Verification items for the finished model (mm, model axes). A direction names the side the tool comes from. Round coordinates to 2 decimals unless told otherwise and drop trailing zeros. Order: outer loops, then holes, each group sorted by start corner. A loop starts at its lowest first (then second) coordinate and runs counter-clockwise, first axis right, second up. Notation, with made-up numbers: (89.25, -11) -> (140.25, -11) arc R30 cw to (140.25, 14) -> close; hole circle Ø9 at (81.5, -12.5). An arc over 180 degrees is marked (long way). Answer in a Markdown table with one row per item. Add a question column.
```python
from build123d import *

# Parameters (mm, degrees)
F0_R     = 1.1684
F1_DEPTH = 4.5085
F3_DEPTH = 4.953
F5_DEPTH = 4.4069
F6_R     = 0.254
F7_DEPTH = 3.81


with BuildPart() as f1:
    # F0 (on Top) → F1 (new body, symmetric)
    with BuildSketch(Plane.XY):
        with BuildLine():
            Line((8.3947, 3.937), (-8.3947, 3.937))
            ThreePointArc((-8.3947, 3.937), (-9.508252, 3.475752), (-9.9695, 2.3622))
            Line((-9.9695, 2.3622), (-9.9695, -2.3622))
            ThreePointArc((-9.9695, -2.3622), (-9.508252, -3.475752), (-8.3947, -3.937))
            Line((-8.3947, -3.937), (8.3947, -3.937))
            ThreePointArc((8.3947, -3.937), (9.508252, -3.475752), (9.9695, -2.3622))
            Line((9.9695, -2.3622), (9.9695, 2.3622))
            ThreePointArc((9.9695, 2.3622), (9.508252, 3.475752), (8.3947, 3.937))
        make_face()
        with Locations((-7.1755, 0)):
            Circle(F0_R, mode=Mode.SUBTRACT)
        with Locations((7.1755, 0)):
            Circle(F0_R, mode=Mode.SUBTRACT)
    extrude(amount=F1_DEPTH, both=True)

    # F2 (on face) → F3 (join)
    with BuildSketch(Plane.XY.offset(4.5085)):
        with BuildLine():
            Line((-3.70192, -3.2893), (3.703378, -3.2893))
            ThreePointArc((3.703378, -3.2893), (5.060271, -2.513771), (5.080729, -0.951022))
            Line((5.080729, -0.951022), (3.292639, 2.274778))
            ThreePointArc((3.292639, 2.274778), (2.714559, 2.868194), (1.915288, 3.0861))
            Line((1.915288, 3.0861), (-1.91383, 3.0861))
            ThreePointArc((-1.91383, 3.0861), (-2.713101, 2.868194), (-3.291181, 2.274778))
            Line((-3.291181, 2.274778), (-5.079271, -0.951022))
            ThreePointArc((-5.079271, -0.951022), (-5.058814, -2.513771), (-3.70192, -3.2893))
        make_face()
    extrude(amount=F3_DEPTH)

    # F4 (on face) → F5 (cut)
    with BuildSketch(Plane.XY.offset(9.4615)):
        with BuildLine():
            Line((1.728266, 2.7686), (-1.726808, 2.7686))
            ThreePointArc((-1.726808, 2.7686), (-2.52608, 2.550694), (-3.104159, 1.957278))
            Line((-3.104159, 1.957278), (-4.791127, -1.086092))
            ThreePointArc((-4.791127, -1.086092), (-4.774629, -2.346374), (-3.68036, -2.9718))
            Line((-3.68036, -2.9718), (3.681817, -2.9718))
            ThreePointArc((3.681817, -2.9718), (4.776086, -2.346374), (4.792584, -1.086092))
            Line((4.792584, -1.086092), (3.105617, 1.957278))
            ThreePointArc((3.105617, 1.957278), (2.527537, 2.550694), (1.728266, 2.7686))
        make_face()
    extrude(amount=-F5_DEPTH, mode=Mode.SUBTRACT)

    # F6 (on face) → F7 (join)
    with BuildSketch(Plane(origin=(0, 0, -4.5085), x_dir=(1, 0, 0), z_dir=(0, 0, -1))):
        with Locations((-3.7973, 0.9525)):
            Circle(F6_R)
        with Locations((-1.8923, 0.9525)):
            Circle(F6_R)
        with Locations((0.0127, 0.9525)):
            Circle(F6_R)
        with Locations((1.9177, 0.9525)):
            Circle(F6_R)
        with Locations((3.8227, 0.9525)):
            Circle(F6_R)
        with Locations((-2.8448, -0.9525)):
            Circle(F6_R)
        with Locations((-0.9398, -0.9525)):
            Circle(F6_R)
        with Locations((0.9652, -0.9525)):
            Circle(F6_R)
        with Locations((2.8702, -0.9525)):
            Circle(F6_R)
    extrude(amount=F7_DEPTH)


solid = f1.part
```
1) Cross-section at B-B, the plane y = 0. Record the boundary of the cut face in (x, z), and give its area (3 significant figures).
2) Thickness scan on L1, parallel to X at y = 0.5, z = -4; L2, parallel to X at y = -0.75, z = 1.5; L3, parallel to Z at x = -8.25, y = -3. Record the ranges inside material, lowest first. Write a range as [from, to].
3) Draft check along X on faces 1 (the face through (0, -3.937, 0)), 2 (the face through (9.496, -3.488, 0.063)), 3 (the face through (0, 2.769, 7)). Enter one of: +X half, -X half, draft (parallel to the pull), parting line (faces both ways), or undercut.
4) Tool access check on faces 4 (the face through (0, 3.086, 7)), 5 (the face through (-3.936, 0.457, 7.289)), 6 (the face through (0, -3.289, 7)). Record the directions out of +Z, -Z, +X, -X, +Y, -Y that give a thin tool (end or side, any length) a straight path to the whole face; none if there is none.
5) Cross-section at C-C, the plane z = -5.5. Give the number of separate pieces and of enclosed holes in the cut face, and give its area (3 significant figures).
6) Depth check by flat-ended pin: P1, Ø3.5, axis at x = -7.18, y = 0, coming from the +Z side; P2, Ø4, axis at x = 1.5, z = -5.5, coming from the +Y side; P3, Ø3.5, axis at x = -0.5, z = 7.5, coming from the +Y side; P4, Ø3, axis at x = -0.5, z = 7.5, coming from the -Y side. Enter the tip coordinate at first touch or a pass-through.
7) Cross-section at A-A, the plane z = 2.25. Record the boundary of the cut face in (x, y), and give its area (3 significant figures).
Results below:
| question | item | result |
|---|---|---|
| 1 | outline | (-9.97, -4.51) -> (-8.34, -4.51) -> (-8.34, 4.51) -> (-9.97, 4.51) -> close; (-6.01, -4.51) -> (6.01, -4.51) -> (6.01, 4.51) -> (4.55, 4.51) -> (4.55, 9.46) -> (4.19, 9.46) -> (4.19, 5.05) -> (-4.19, 5.05) -> (-4.19, 9.46) -> (-4.55, 9.46) -> (-4.55, 4.51) -> (-6.01, 4.51) -> close; (8.34, -4.51) -> (9.97, -4.51) -> (9.97, 4.51) -> (8.34, 4.51) -> close |
| 1 | area | 146 mm² |
| 2 | L1 | [-9.97, -8.23], [-6.12, 6.12], [8.23, 9.97] |
| 2 | L2 | [-9.97, -8.07], [-6.28, 6.28], [8.07, 9.97] |
| 2 | L3 | [-4.51, 4.51] |
| 3 | face 1 | draft |
| 3 | face 2 | +X half |
| 3 | face 3 | undercut |
| 4 | face 4 | +Z, +X, -X, +Y |
| 4 | face 5 | +Z |
| 4 | face 6 | +Z, +X, -X, -Y |
| 5 | separate pieces | 9 |
| 5 | enclosed holes | 0 |
| 5 | area | 1.82 mm² |
| 6 | P1 | z = 4.51 |
| 6 | P2 | y = 3.94 |
| 6 | P3 | y = 3.09 |
| 6 | P4 | y = -3.29 |
| 7 | outline | (-9.97, -2.36) arc R1.57 ccw to (-8.39, -3.94) -> (8.39, -3.94) arc R1.57 ccw to (9.97, -2.36) -> (9.97, 2.36) arc R1.57 ccw to (8.39, 3.94) -> (-8.39, 3.94) arc R1.57 ccw to (-9.97, 2.36) -> close; hole circle Ø2.34 at (-7.18, 0); hole circle Ø2.34 at (7.18, 0) |
| 7 | area | 146 mm² |
